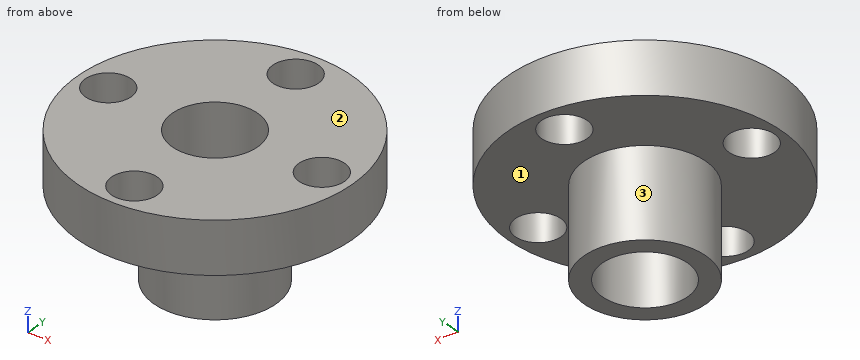
from build123d import *

# Parameters (mm, degrees)
SKETCH2_R                = 225
SKETCH2_R_2              = 100
BOSS_EXTRUDE1_DEPTH      = 85
BOSS_EXTRUDE2_DEPTH      = 145
BOSS_EXTRUDE2_DEPTH_BACK = 85
SKETCH3_R                = 100
SKETCH4_R                = 70
CUT_EXTRUDE1_DEPTH       = 315
SKETCH5_R                = 37.5
CUT_EXTRUDE2_DEPTH       = 85


with BuildPart() as part:
    # Sketch2 → Boss-Extrude1 (new body)
    with BuildSketch(Plane.XY):
        Circle(SKETCH2_R)
        Circle(SKETCH2_R_2, mode=Mode.SUBTRACT)
    extrude(amount=BOSS_EXTRUDE1_DEPTH)

    # Sketch3 → Boss-Extrude2 (add, two sides: drawn at the far end of the back side and taken through both)
    with BuildSketch(Plane(origin=(0, 0, 0), x_dir=(-1, 0, 0), z_dir=(0, 0, -1)).offset(-BOSS_EXTRUDE2_DEPTH_BACK)):
        Circle(SKETCH3_R)
    extrude(amount=BOSS_EXTRUDE2_DEPTH + BOSS_EXTRUDE2_DEPTH_BACK)

    # Sketch4 → Cut-Extrude1 (cut)
    with BuildSketch(Plane(origin=(0, 0, -145), x_dir=(-1, 0, 0), z_dir=(0, 0, -1))):
        Circle(SKETCH4_R)
    extrude(amount=-CUT_EXTRUDE1_DEPTH, mode=Mode.SUBTRACT)

    # Sketch5 → Cut-Extrude2 (cut)
    with BuildSketch(Plane.XY.offset(85)):
        with Locations((175, 0)):
            Circle(SKETCH5_R)
        with Locations((0, 175)):
            Circle(SKETCH5_R)
        with Locations((-175, 0)):
            Circle(SKETCH5_R)
        with Locations((0, -175)):
            Circle(SKETCH5_R)
    extrude(amount=-CUT_EXTRUDE2_DEPTH, mode=Mode.SUBTRACT)


solid = part.part
CAD build for the part. Positions are in the model's coordinates, mm. Face numbers are marked on the shaded views. Round coordinates to 2 decimals unless told otherwise and drop trailing zeros. Loops run counter-clockwise (first coordinate to the right, second up) from the corner with the lowest first, then second, coordinate; pieces in that order, holes last. Notation, with made-up numbers: M -32,9 L 1,9 A29 ccw 1,39 Z; hole C 71,30.5 d7. An arc over 180 degrees is marked long. One line per question, with ' | ' between items. Start each with the question number.
Item 1: Two-plate mould, pull along Z, no slides. Class the marked faces 1, 2 and 3: pulls with the +Z half, pulls with the -Z half, needs draft (parallel to the pull), parting line crosses it, or undercut.
Item 2: Cut at A-A, the plane x = 6.5. Write the cut outline in (y, z).
Item 3: Pin check, flat tips, straight feed: pin 1 Ø3 at (y, z) = (68.5, 56) entering from -X; pin 2 Ø10 at (x, y) = (-149, 89.5) entering from -Z; pin 3 Ø5 at (x, z) = (-38.5, 47) entering from -Y. Stop position of each tip, or through.
Item 4: Cut at C-C, the plane x = -148.5. Write the cut outline in (y, z), plus the area to 3 significant figures.
Item 5: Cut at D-D, the plane z = -109. Write the cut outline in (x, y), plus the area to 3 significant figures.
Item 6: Cut at B-B, the plane y = 175. Write the cut outline in (x, z).
Item 7: Wall check: line 1 (Y direction, x = 9, z = 21); line 2 (Y direction, x = -34, z = 19); line 3 (Y direction, x = 0, z = -61). Give the ranges that are in metal, low to high.
Responses:
1) face 1: pulls with the -Z half | face 2: pulls with the +Z half | face 3: needs draft
2) outline: M -224.91,0 L -211.93,0 L -211.93,85 L -224.91,85 Z; M -138.07,0 L -99.79,0 L -99.79,-145 L -69.7,-145 L -69.7,85 L -138.07,85 Z; M 69.7,-145 L 99.79,-145 L 99.79,0 L 138.07,0 L 138.07,85 L 69.7,85 Z; M 211.93,0 L 224.91,0 L 224.91,85 L 211.93,85 Z
3) pin 1: stops at x = -214.79 | pin 2: stops at z = 0 | pin 3: stops at y = -222.1
4) outline: M -169.03,0 L -26.53,0 L -26.53,85 L -169.03,85 Z; M 26.53,0 L 169.03,0 L 169.03,85 L 26.53,85 Z | area: 24,200 mm²
5) outline: C 0,0 d200; hole C 0,0 d140 | area: 16,000 mm²
6) outline: M -141.42,0 L -37.5,0 L -37.5,85 L -141.42,85 Z; M 37.5,0 L 141.42,0 L 141.42,85 L 37.5,85 Z
7) line 1: y = -224.82 to -211.4, -138.6 to -69.42, 69.42 to 138.6, 211.4 to 224.82 | line 2: y = -222.42 to -190.82, -159.18 to -61.19, 61.19 to 159.18, 190.82 to 222.42 | line 3: y = -100 to -70, 70 to 100
